from build123d import *

# Parameters (mm, degrees)
F1_DEPTH  = 3.175
F2_R      = 2.54
F3_R      = 1.27
F1_FACE_W = 3.302
F1_FACE_H = 3.175
F4_DEPTH  = 1.143


with BuildPart() as f1:
    # F0 (on Top) → F1 (new body)
    with BuildSketch(Plane.XY):
        Polygon((9.525, 44.45), (-9.525, 44.45), (-9.525, 34.29), (0.127, 34.29), (0.127, 30.988), (-9.525, 30.988), (-9.525, -30.988), (0.127, -30.988), (0.127, -34.29), (-9.525, -34.29), (-9.525, -44.45), (9.525, -44.45), align=None)
    extrude(amount=F1_DEPTH)

    # F2
    f2_edges = [f1.edges().sort_by_distance(p)[0] for p in [
        (-9.525, 44.45, 1.5875),
        (9.525, 44.45, 1.5875),
        (9.525, -44.45, 1.5875),
        (-9.525, -44.45, 1.5875),
    ]]
    fillet(f2_edges, radius=F2_R)

    # F3
    f3_edges = [f1.edges().sort_by_distance(p)[0] for p in [
        (-9.525, 34.29, 1.5875),
        (-9.525, -30.988, 1.5875),
        (-9.525, 30.988, 1.5875),
        (-9.525, -34.29, 1.5875),
    ]]
    fillet(f3_edges, radius=F3_R)

    # F1_face (on face) → F4 (cut)
    with BuildSketch(Plane(origin=(0.127, 32.639, 1.5875), x_dir=(0, -1, 0), z_dir=(-1, 0, 0))):
        Rectangle(F1_FACE_W, F1_FACE_H)
        with Locations((65.278, 0)):
            Rectangle(F1_FACE_W, F1_FACE_H)
    extrude(amount=-F4_DEPTH, mode=Mode.SUBTRACT)


solid = f1.part
CAD build for the part. Positions are in the model's coordinates, mm. A direction names the side the tool comes from. Round coordinates to 2 decimals unless told otherwise and drop trailing zeros. Write each loop counter-clockwise with the first axis right and the second up, starting at its lowest first coordinate (ties: lowest second). Pieces come first, ordered by that corner, then holes.
(1) Slice it at A-A, the plane x = -0.5. Write the cut outline in (y, z) (3 decimals).
(2) Mould opens along Y. For faces 1 (the face through (-3, -34.29, 2)), 2 (the face through (-4, -30.988, 2)), 3 (the face through (0, 1, 3.175)), 4 (the face through (-8.801, -43.686, 1.61)) say: pulls with the +Y half, pulls with the -Y half, needs draft (parallel to the pull), parting line crosses it, or undercut.
(3) Drop a flat-ended pin along its axis: P1, Ø1.6, axis at y = -32.5, z = 2, coming from the -X side. Give the stop position or say it passes through.
(4) Slice it at B-B, the plane z = 0.9. Write the cut outline in (x, y) (3 decimals).
(5) 3-axis set-ups, long thin cutter, end or side, ignore diameter. For faces 5 (the face through (1.27, 33, 2)), 6 (the face through (-8.761, 43.726, 1.61)): which of +Z, -Z, +X, -X, +Y, -Y reach the whole face in a straight line?
(6) Probe line 1 along Y through (x, z) = (-6.25, 0.9); line 2 along X through (y, z) = (-35.5, 2.3) (3 decimals); line 3 along Y through (x, z) = (-8.5, 0.35). List the from-to ranges inside material, lowest first.
From the geometry:
1. outline: (-44.45, 0) - (-34.29, 0) - (-34.29, 3.175) - (-44.45, 3.175) - close; (-30.988, 0) - (30.988, 0) - (30.988, 3.175) - (-30.988, 3.175) - close; (34.29, 0) - (44.45, 0) - (44.45, 3.175) - (34.29, 3.175) - close
2. face 1: undercut
2. face 2: undercut
2. face 3: needs draft
2. face 4: pulls with the -Y half
3. P1: stops at x = 1.27
4. outline: (-9.525, -41.91) arc R2.54 ccw to (-6.985, -44.45) - (6.985, -44.45) arc R2.54 ccw to (9.525, -41.91) - (9.525, 41.91) arc R2.54 ccw to (6.985, 44.45) - (-6.985, 44.45) arc R2.54 ccw to (-9.525, 41.91) - (-9.525, 35.56) arc R1.27 ccw to (-8.255, 34.29) - (1.27, 34.29) - (1.27, 30.988) - (-8.255, 30.988) arc R1.27 ccw to (-9.525, 29.718) - (-9.525, -29.718) arc R1.27 ccw to (-8.255, -30.988) - (1.27, -30.988) - (1.27, -34.29) - (-8.255, -34.29) arc R1.27 ccw to (-9.525, -35.56) - close
5. face 5: +Z, -Z, -X
5. face 6: +Z, -Z, -X, +Y
6. line 1: y = -44.45 to -34.29, -30.99 to 30.99, 34.29 to 44.45
6. line 2: x = -9.524 to 9.525
6. line 3: y = -43.95 to -34.31, -30.96 to 30.96, 34.31 to 43.95
